Check sheet for the modelled part. Datum: model origin and axes. Units: mm. Face numbers are marked on the shaded views. A direction names the side the tool comes from. Give positions to 0.01 mm unless a question says otherwise; leave off trailing zeros. Write each loop counter-clockwise with the first axis right and the second up, starting at its lowest first coordinate (ties: lowest second). Pieces come first, ordered by that corner, then holes. Notation, with made-up numbers: (87.25, 72.25) -> (146.25, 72.25) arc R27 cw to (146.25, 104.25) -> close; hole circle Ø9 at (28, -21.5). An arc over 180 degrees is marked (long way). Use a Markdown table: item, result. Add a question column.
1. Cross-section at D-D (z = 46.25). Enter the section's corners in (x, y).
2. Cross-section at A-A (z = -47). Enter the section's corners in (x, y).
3. Cross-section at C-C (x = 6). Enter the section's corners in (y, z) (3 decimals).
4. Cross-section at B-B (z = -6.5). Enter the section's corners in (x, y), then the cut area to 3 significant figures.
5. Set-up check for the marked faces 1 and 2: record each of +Z, -Z, +X, -X, +Y, -Y from which the full face is reachable in a straight line by a thin tool's end or side.
6. Gauge pin test, flat ends, axial feed: P1, Ø4, axis at y = 40.1, z = -40, coming from the -X side; P2, Ø3, axis at x = 11, y = -1.5, coming from the -Z side; P3, Ø5, axis at x = 6, y = 23.5, coming from the -Z side; P4, Ø1, axis at x = 19, y = -7.5, coming from the +Z side. Record the tip position at first contact, or that the pin passes through.
7. Scan lines: probe 1 along Y at (x, z) = (24.4, -60); probe 2 along Y at (x, z) = (1.25, 23); probe 3 along X at (y, z) = (36, -42.5). Record each from-to range of solid material in increasing order. Write a range as [from, to].
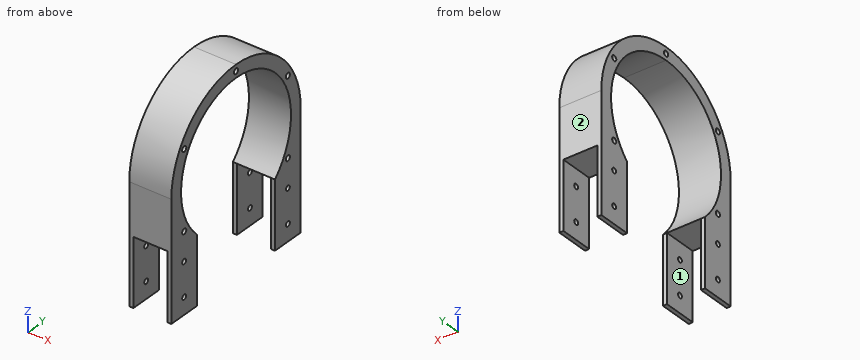
from build123d import *

# Parameters (mm, degrees)
SKETCH_1_R          = 1.6
EXTRUDE_1_DEPTH     = 25
SKETCH_2_W          = 2.43
SKETCH_2_H          = 19.896013553
EXTRUDE_2_DEPTH     = 40
SKETCH_4_R          = 1.5
CUT_EXTRUDE_4_DEPTH = 90.582364336


with BuildPart() as part:
    # 草图1 → 凸台-拉伸1 (new body)
    # profile 1 of 2: a face of its own
    with BuildSketch(Plane(origin=(0, 0, 0), x_dir=(0, 0, -1), z_dir=(1, 0, 0))):
        with BuildLine():
            ThreePointArc((-47.85, 0), (-46.25, 1.6), (-44.65, 0))
            Line((-44.65, 0), (-42.5, 0))
            ThreePointArc((-42.5, 0), (-16.298006013, 39.25079617), (30, 30.103986447))
            Line((30, 30.103986447), (30, 50))
            Line((30, 50), (0, 50))
            ThreePointArc((0, 50), (-35.355339059, 35.355339059), (-50, 0))
            Line((-50, 0), (-47.85, 0))
        make_face()
        with Locations((-23.125, 40.053674925)):
            Circle(SKETCH_1_R, mode=Mode.SUBTRACT)
        with Locations((23.125, 40.053674925)):
            Circle(SKETCH_1_R, mode=Mode.SUBTRACT)
    # profile 2 of 2: a face of its own
    with BuildSketch(Plane(origin=(0, 0, 0), x_dir=(0, 0, -1), z_dir=(1, 0, 0))):
        with BuildLine():
            Line((-42.5, 0), (-44.65, 0))
            ThreePointArc((-44.65, 0), (-46.25, -1.6), (-47.85, 0))
            Line((-47.85, 0), (-50, 0))
            ThreePointArc((-50, 0), (-35.355339059, -35.355339059), (0, -50))
            Line((0, -50), (30, -50))
            Line((30, -50), (30, -30.103986447))
            ThreePointArc((30, -30.103986447), (-16.298006013, -39.25079617), (-42.5, 0))
        make_face()
        with Locations((-23.125, -40.053674925)):
            Circle(SKETCH_1_R, mode=Mode.SUBTRACT)
        with Locations((23.125, -40.053674925)):
            Circle(SKETCH_1_R, mode=Mode.SUBTRACT)
    extrude(amount=EXTRUDE_1_DEPTH)

    # 草图2 → 凸台-拉伸2 (add)
    with BuildSketch(Plane(origin=(0, 0, -30), x_dir=(-1, 0, 0), z_dir=(0, 0, -1))):
        with Locations((-23.785, 40.051993223)):
            Rectangle(SKETCH_2_W, SKETCH_2_H)
        with Locations((-1.215, 40.051993223)):
            Rectangle(SKETCH_2_W, SKETCH_2_H)
        with Locations((-1.215, -40.051993223)):
            Rectangle(SKETCH_2_W, SKETCH_2_H)
        with Locations((-23.785, -40.051993223)):
            Rectangle(SKETCH_2_W, SKETCH_2_H)
    extrude(amount=EXTRUDE_2_DEPTH)

    # 草图4 → 切除-拉伸4 (cut, through all)
    with BuildSketch(Plane(origin=(25, 0, 0), x_dir=(0, 0, -1), z_dir=(1, 0, 0))):
        with Locations((60, -40.103986447)):
            Circle(SKETCH_4_R)
        with Locations((40, -40.103986447)):
            Circle(SKETCH_4_R)
        with Locations(Location((40, 40.103986447, 0), (0, 0, 270))):
            Circle(SKETCH_4_R)
        with Locations(Location((60, 40.103986447, 0), (0, 0, 270))):
            Circle(SKETCH_4_R)
    extrude(amount=-CUT_EXTRUDE_4_DEPTH, mode=Mode.SUBTRACT)


solid = part.part
Worked answers:
| question | item | result |
|---|---|---|
| 1 | outline | (0, -19) -> (25, -19) -> (25, -1.6) -> (0, -1.6) -> close; (0, 1.6) -> (25, 1.6) -> (25, 19) -> (0, 19) -> close |
| 2 | outline | (0, -50) -> (2.43, -50) -> (2.43, -30.1) -> (0, -30.1) -> close; (0, 30.1) -> (2.43, 30.1) -> (2.43, 50) -> (0, 50) -> close; (22.57, -50) -> (25, -50) -> (25, -30.1) -> (22.57, -30.1) -> close; (22.57, 30.1) -> (25, 30.1) -> (25, 50) -> (22.57, 50) -> close |
| 3 | outline | (-50, -30) -> (-30.104, -30) arc R42.5 cw (long way) to (30.104, -30) -> (50, -30) -> (50, 0) arc R50 ccw to (-50, 0) -> close; hole circle Ø3.2 at (-40.054, -23.125); hole circle Ø3.2 at (-40.054, 23.125); hole circle Ø3.2 at (0, 46.25); hole circle Ø3.2 at (40.054, -23.125); hole circle Ø3.2 at (40.054, 23.125) |
| 4 | outline | (0, -50) -> (25, -50) -> (25, -42) -> (0, -42) -> close; (0, 42) -> (25, 42) -> (25, 50) -> (0, 50) -> close |
| 4 | area | 400 mm² |
| 5 | face 1 | -Z, +Y, -Y |
| 5 | face 2 | +Z, -Z, +X, -X, +Y |
| 6 | P1 | stops at x = 0 |
| 6 | P2 | stops at z = 42.39 |
| 6 | P3 | stops at z = 33.62 |
| 6 | P4 | stops at z = 49.51 |
| 7 | probe 1 | y = [-50, -41.6], [-38.6, -30.1], [30.1, 38.6], [41.6, 50] |
| 7 | probe 2 | y = [-44.4, -41.65], [-38.46, -35.74], [35.74, 38.46], [41.65, 44.4] |
| 7 | probe 3 | x = [0, 2.43], [22.57, 25] |
